Can you work these out from the model? Positions are in its coordinate system, mm. Face numbers are marked on the shaded views. Round coordinates to 2 decimals unless told otherwise and drop trailing zeros. Loops run counter-clockwise (first coordinate to the right, second up) from the corner with the lowest first, then second, coordinate; pieces in that order, holes last.
(1) If I drill on line 1 along Y through (x, z) = (0, 0); line 2 along Y through (x, z) = (-3.5, -0.5); line 3 along X through (y, z) = (-1.25, 1.25), over which ranges is the centre line in solid material (lowest first)?
(2) Thinking about a two-plate mould opening in Y: for the marked faces 1, 2 and 3, which applies, released by +Y, released by -Y, zero draft, split by the parting line, or undercut?
(3) I want a section at A-A on z = -1. Write out the boundary of the cut face in (x, y), plus the area to 3 significant figures.
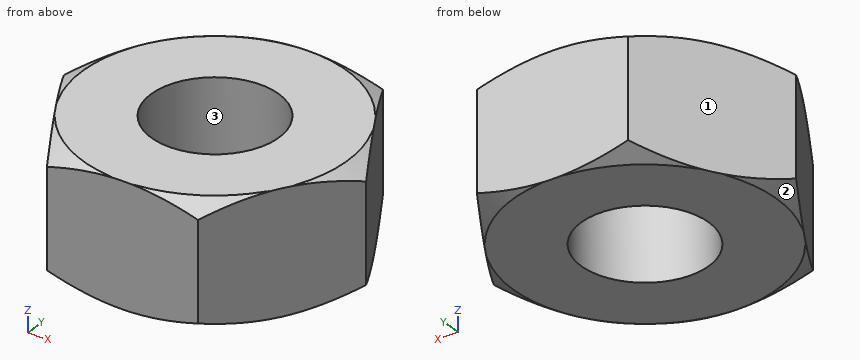
Solid Edge part; units mm, degrees
sketch "Sketch1" plane through (0, 0, 0) normal (0, 0, 1) x (1, 0, 0)
  line L0 (-5, -8.6603) -> (5, -8.6603)
  line L1 (5, -8.6603) -> (10, 0)
  line L2 (10, 0) -> (5, 8.6603)
  line L3 (5, 8.6603) -> (-5, 8.6603)
  line L4 (-5, 8.6603) -> (-10, 0)
  line L5 (-10, 0) -> (-5, -8.6603)
extrude "Protrusion1" add sketch "Sketch1" along normal mid plane 8
hole "Hole_1" at (0, 0, 4) direction (0, 0, -1) diameter 8.376 end through all
sketch "Sketch2" plane through (0, 0, 0) normal (1, 0, 0) x (0, 1, 0)
  line L0 (8.6603, -4) -> (27.7764, 7.0367)
revolve "RevolvedCutout1" cut sketch "Sketch2" angle 360 about axis through (0, 0, -57) along (0, 0, 1) material side at (0, 18.2434, 1.475)
mirror "Mirror1" about plane through (0, 0, 0) normal (0, 0, 1) of "RevolvedCutout1"
properties part number "7" material "Fe 410 W"
Filled sheet:
1. line 1: y = -8.66 to -4.19, 4.19 to 8.66
1. line 2: y = -8.66 to -2.3, 2.3 to 8.66
1. line 3: x = -9.28 to -4, 4 to 9.28
2. face 1: released by +Y
2. face 2: split by the parting line
2. face 3: undercut
3. outline: (-10, 0) - (-5, -8.66) - (5, -8.66) - (10, 0) - (5, 8.66) - (-5, 8.66) - close; hole circle Ø8.38 at (0, 0)
3. area: 205 mm2
